Design review of the part built by this model. Coordinates are the model's own, in mm. Face numbers are marked on the shaded views. Round coordinates to 2 decimals unless told otherwise and drop trailing zeros. Loops run counter-clockwise (first coordinate to the right, second up) from the corner with the lowest first, then second, coordinate; pieces in that order, holes last. Notation, with made-up numbers: (58, 31) -> (75, 31) arc R26 cw to (75, 49) -> close; hole circle Ø6 at (55, 0). An arc over 180 degrees is marked (long way). Use a Markdown table: item, result. Add a question column.
from build123d import *

# Parameters (mm, degrees)
F1_DEPTH = 50
F2_R     = 2.5
F3_DEPTH = 25
F4_R     = 1


with BuildPart() as f1:
    # F0 (on Front) → F1 (new body, symmetric)
    with BuildSketch(Plane.XZ):
        with BuildLine():
            Line((11.7, 7.5), (0, 7.5))
            Line((0, 7.5), (-11.7, 7.5))
            ThreePointArc((-11.7, 7.5), (-12.972792, 6.972792), (-13.5, 5.7))
            Line((-13.5, 5.7), (-13.5, 1.8))
            ThreePointArc((-13.5, 1.8), (-13.734315, 1.234315), (-14.3, 1))
            Line((-14.3, 1), (-17.5, 1))
            Line((-17.5, 1), (-17.5, 0))
            Line((-17.5, 0), (-14.3, 0))
            ThreePointArc((-14.3, 0), (-13.027208, 0.527208), (-12.5, 1.8))
            Line((-12.5, 1.8), (-12.5, 5.7))
            ThreePointArc((-12.5, 5.7), (-12.265685, 6.265685), (-11.7, 6.5))
            Line((-11.7, 6.5), (0, 6.5))
            Line((0, 6.5), (11.7, 6.5))
            ThreePointArc((11.7, 6.5), (12.265685, 6.265685), (12.5, 5.7))
            Line((12.5, 5.7), (12.5, 1.8))
            ThreePointArc((12.5, 1.8), (13.027208, 0.527208), (14.3, 0))
            Line((14.3, 0), (17.5, 0))
            Line((17.5, 0), (17.5, 1))
            Line((17.5, 1), (14.3, 1))
            ThreePointArc((14.3, 1), (13.734315, 1.234315), (13.5, 1.8))
            Line((13.5, 1.8), (13.5, 5.7))
            ThreePointArc((13.5, 5.7), (12.972792, 6.972792), (11.7, 7.5))
        make_face()
    extrude(amount=F1_DEPTH, both=True)

    # F2 (on face) → F3 (cut)
    with BuildSketch(Plane.XY.offset(7.5)):
        with Locations((0, 30)):
            Circle(F2_R)
        with Locations((0, -30)):
            Circle(F2_R)
    extrude(amount=-F3_DEPTH, mode=Mode.SUBTRACT)

    # F4
    f4_edges = [f1.edges().sort_by_distance(p)[0] for p in [
        (17.5, 50, 0.5),
        (-17.5, 50, 0.5),
        (17.5, -50, 0.5),
        (-17.5, -50, 0.5),
    ]]
    fillet(f4_edges, radius=F4_R)


solid = f1.part
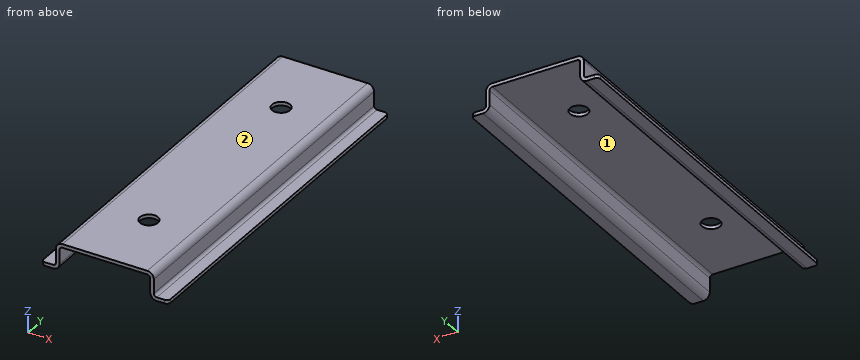
1. Consider section A-A on y = -30. State the section outline as (x, z) points, plus the area to 3 significant figures.
2. To check wall thickness, follow probe 1 along Y at (x, z) = (0, 6.9); probe 2 along X at (y, z) = (-37.5, 2); probe 3 along Y at (x, z) = (1, 7). State the ranges of each line that lie inside material, in increasing order. Write a range as from..to.
3. Mouldability with a two-part tool opening along X and no side actions: class the marked faces 1 and 2 as +X half, -X half, draft (parallel to the pull), parting line (faces both ways), or undercut.
4. Consider section B-B on x = 0. State the section outline as (y, z) points, plus the area to 3 significant figures.
5. Consider section C-C on z = 4. State the section outline as (x, y) points, plus the area to 3 significant figures.
6. Consider section D-D on y = 41. State the section outline as (x, z) points.
7. Insertion check: P1, Ø12, axis at x = 5.5, y = 2.5, coming from the -Z side; P2, Ø1.2, axis at y = -18.5, z = 4, coming from the +X side; P3, Ø1.6, axis at x = 15.5, y = 17, coming from the +Z side. Each pin has a flat end and moves straight along its axis. Give the tip position at first contact, or say it passes through.
Verdict:
| question | item | result |
|---|---|---|
| 1 | outline | (-17.5, 0) -> (-14.3, 0) arc R1.8 ccw to (-12.5, 1.8) -> (-12.5, 5.7) arc R0.8 cw to (-11.7, 6.5) -> (-2.5, 6.5) -> (-2.5, 7.5) -> (-11.7, 7.5) arc R1.8 ccw to (-13.5, 5.7) -> (-13.5, 1.8) arc R0.8 cw to (-14.3, 1) -> (-17.5, 1) -> close; (2.5, 6.5) -> (11.7, 6.5) arc R0.8 cw to (12.5, 5.7) -> (12.5, 1.8) arc R1.8 ccw to (14.3, 0) -> (17.5, 0) -> (17.5, 1) -> (14.3, 1) arc R0.8 cw to (13.5, 1.8) -> (13.5, 5.7) arc R1.8 ccw to (11.7, 7.5) -> (2.5, 7.5) -> close |
| 1 | area | 40.8 mm² |
| 2 | probe 1 | y = -50..-32.5, -27.5..27.5, 32.5..50 |
| 2 | probe 2 | x = -13.5..-12.5, 12.5..13.5 |
| 2 | probe 3 | y = -50..-32.29, -27.71..27.71, 32.29..50 |
| 3 | face 1 | undercut |
| 3 | face 2 | draft |
| 4 | outline | (-50, 6.5) -> (-32.5, 6.5) -> (-32.5, 7.5) -> (-50, 7.5) -> close; (-27.5, 6.5) -> (27.5, 6.5) -> (27.5, 7.5) -> (-27.5, 7.5) -> close; (32.5, 6.5) -> (50, 6.5) -> (50, 7.5) -> (32.5, 7.5) -> close |
| 4 | area | 90.0 mm² |
| 5 | outline | (-13.5, -50) -> (-12.5, -50) -> (-12.5, 50) -> (-13.5, 50) -> close; (12.5, -50) -> (13.5, -50) -> (13.5, 50) -> (12.5, 50) -> close |
| 5 | area | 200 mm² |
| 6 | outline | (-17.5, 0) -> (-14.3, 0) arc R1.8 ccw to (-12.5, 1.8) -> (-12.5, 5.7) arc R0.8 cw to (-11.7, 6.5) -> (11.7, 6.5) arc R0.8 cw to (12.5, 5.7) -> (12.5, 1.8) arc R1.8 ccw to (14.3, 0) -> (17.5, 0) -> (17.5, 1) -> (14.3, 1) arc R0.8 cw to (13.5, 1.8) -> (13.5, 5.7) arc R1.8 ccw to (11.7, 7.5) -> (-11.7, 7.5) arc R1.8 ccw to (-13.5, 5.7) -> (-13.5, 1.8) arc R0.8 cw to (-14.3, 1) -> (-17.5, 1) -> close |
| 7 | P1 | stops at z = 6.5 |
| 7 | P2 | stops at x = 13.5 |
| 7 | P3 | stops at z = 1 |
